Here's the drawing with two shaded views (mm, measured from the low corner). I have some questions. A direction names the side the tool comes from. Round coordinates to 2 decimals unless told otherwise and drop trailing zeros. Loops run counter-clockwise (first coordinate to the right, second up) from the corner with the lowest first, then second, coordinate; pieces in that order, holes last. Notation, with made-up numbers: (49.5, 26) -> (92.5, 26) arc R26 cw to (92.5, 50) -> close; hole circle Ø5 at (71.5, -24). An arc over 180 degrees is marked (long way). Write item = value, one per line.
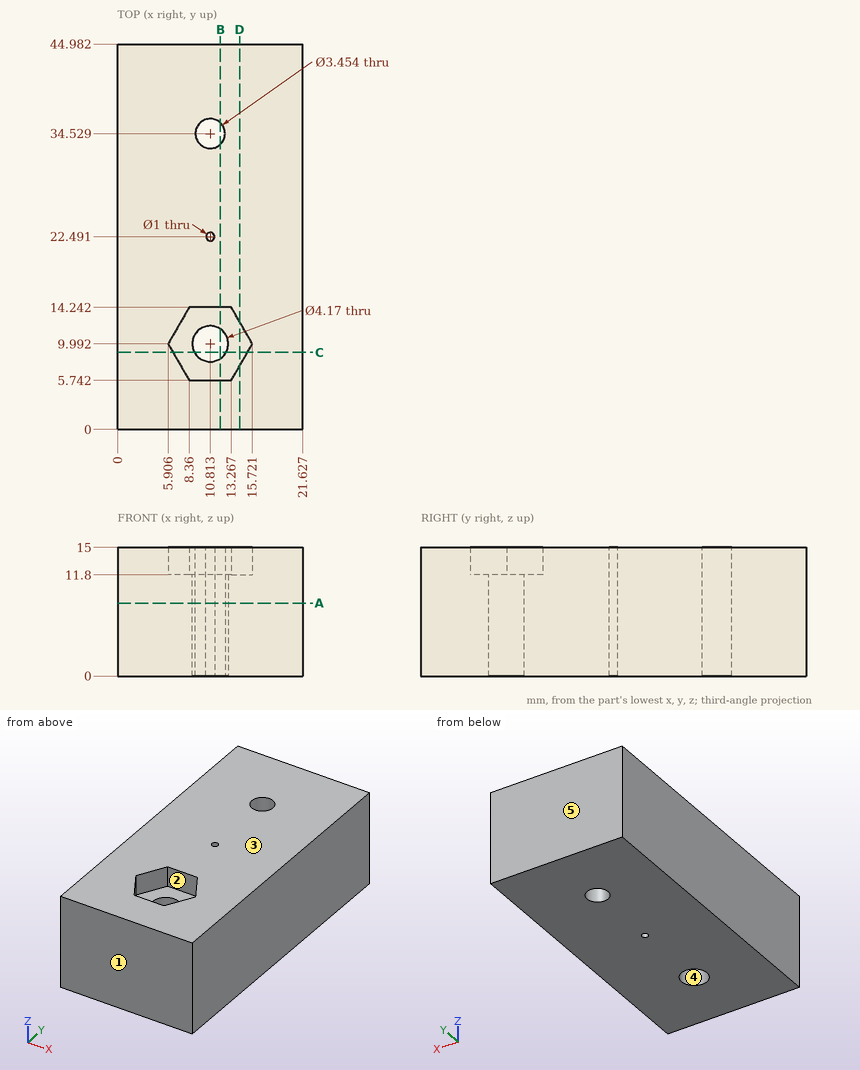
1. Suppose I cut it at C-C, the plane y = 9. List the corners of the cut face in (x, z) for me, and give its area (3 significant figures).
Entries:
outline = (0, 0) -> (8.98, 0) -> (8.98, 11.8) -> (6.48, 11.8) -> (6.48, 15) -> (0, 15) -> close; (12.65, 0) -> (21.63, 0) -> (21.63, 15) -> (15.15, 15) -> (15.15, 11.8) -> (12.65, 11.8) -> close
area = 253 mm²
2. For the marked faces 1 and 2, which set-ups out of +Z, -Z, +X, -X, +Y, -Y let a thin tool reach every point of the face, with its end or its side?
Entries:
face_1 = +Z, -Z, +X, -X, -Y
face_2 = +Z
3. Suppose I cut it at B-B, the plane x = 12. List the corners of the cut face in (y, z) for me (1 decimal).
Entries:
outline = (0, 0) -> (8.3, 0) -> (8.3, 11.8) -> (5.7, 11.8) -> (5.7, 15) -> (0, 15) -> close; (11.7, 0) -> (33.3, 0) -> (33.3, 15) -> (14.2, 15) -> (14.2, 11.8) -> (11.7, 11.8) -> close; (35.8, 0) -> (45, 0) -> (45, 15) -> (35.8, 15) -> close
4. We'd pull the mould along Y, two halves only. Please class the marked faces 3, 4 and 5: released by +Y, released by -Y, zero draft, split by the parting line, or undercut.
Entries:
face_3 = zero draft
face_4 = undercut
face_5 = released by +Y
5. I need wall thicknesses on line 1 (Y direction, x = 11.75, z = 8) (1 decimal); line 2 (Y direction, x = 10.5, z = 7.5) (1 decimal); line 3 (Y direction, x = 7.25, z = 12.75) (1 decimal). Which ranges of each line are inside material? Lowest first, please. Write a range as [from, to].
Entries:
line_1 = [0, 8.1], [11.9, 33.1], [36, 45]
line_2 = [0, 7.9], [12.1, 22.1], [22.9, 32.8], [36.2, 45]
line_3 = [0, 7.7], [12.3, 45]
6. Suppose I cut it at D-D, the plane x = 14.25. List the corners of the cut face in (y, z) for me (1 decimal).
Entries:
outline = (0, 0) -> (45, 0) -> (45, 15) -> (12.5, 15) -> (12.5, 11.8) -> (7.4, 11.8) -> (7.4, 15) -> (0, 15) -> close
7. Suppose I cut it at A-A, the plane z = 8.5. List the corners of the cut face in (x, y) for me (1 decimal).
Entries:
outline = (0, 0) -> (21.6, 0) -> (21.6, 45) -> (0, 45) -> close; hole circle Ø4.2 at (10.8, 10); hole circle Ø3.5 at (10.8, 34.5); hole circle Ø1 at (10.8, 22.5)
